Geometry check sheet. Reference: the model listing, model coordinates, mm. Face numbers are marked on the shaded views. A direction names the side the tool comes from. Give positions to 0.01 mm unless a question says otherwise; leave off trailing zeros. Write each loop counter-clockwise with the first axis right and the second up, starting at its lowest first coordinate (ties: lowest second). Pieces come first, ordered by that corner, then holes. Notation, with made-up numbers: (-40, 42) - (19, 42) arc R26 ccw to (19, 78) - close; hole circle Ø4 at (80, -14). An arc over 180 degrees is marked (long way). Write item = value, one per line. Start each with the question number.
(1) Access from +Z, -Z, +X, -X, +Y, -Y to the whole of each face (thin tool, end or side, straight path). Record for the marked faces 4, 5, 6, 7 and 8.
(2) Draft check along X on the marked faces 1, 2 and 3. Enter one of: pulls with the +X half, pulls with the -X half, needs draft (parallel to the pull), parting line crosses it, or undercut.
(3) Section check D-D, the plane z = -0.25. Give the number of separate pieces and of enclosed holes in the cut face, plus the area to 3 significant figures.
(4) Thickness scan on L1, parallel to Y at x = 0, z = 0.5 (3 decimals); L2, parallel to Z at x = -6, y = 10.75 (3 decimals); L3, parallel to Y at x = 0, z = -5 (3 decimals). Record the ranges inside material, lowest first.
(5) Section check A-A, the plane z = -5.5. Enter the section's corners in (x, y) (3 decimals), plus the area to 3 significant figures.
(6) Depth check by flat-ended pin: pin 1 Ø5 at (x, z) = (-13, -7) entering from +Y; pin 2 Ø6.5 at (x, y) = (-2.5, -4.5) entering from +Z (3 decimals); pin 3 Ø5 at (y, z) = (14.5, -2) entering from +X. Enter the tip coordinate at first touch or a pass-through.
(7) Section check B-B, the plane y = 13.5. Enter the section's corners in (x, z) (3 decimals), plus the area to 3 significant figures.
```python
from build123d import *

# Parameters (mm, degrees)
SKETCH1_W           = 38.1
SKETCH1_H           = 19.05
BOSS_EXTRUDE1_DEPTH = 19.05
SKETCH2_R           = 1.5875
CUT_EXTRUDE2_DEPTH  = 19.05
SKETCH3_W           = 16.620070223
SKETCH3_H           = 12.7
CUT_EXTRUDE3_DEPTH  = 19.05
SKETCH4_W           = 12.7
SKETCH4_H           = 12.7
CUT_EXTRUDE4_DEPTH  = 50.8
SKETCH6_W           = 7.660570014
SKETCH6_H           = 3.81
BOSS_EXTRUDE2_DEPTH = 7.62
CUT_EXTRUDE6_DEPTH  = 19.05
SKETCH8_W           = 5.08
SKETCH8_H           = 2.54
BOSS_EXTRUDE3_DEPTH = 2.54
SKETCH9_R           = 0.508
CUT_EXTRUDE7_DEPTH  = 19.05
SKETCH10_W          = 9.525
SKETCH10_H          = 12.7
CUT_EXTRUDE8_DEPTH  = 3.81


with BuildPart() as part:
    # Sketch1 → Boss-Extrude1 (new body)
    with BuildSketch(Plane(origin=(0, 0, 0), x_dir=(1, 0, 0), z_dir=(0, 1, 0))):
        with Locations((-3.175, 0)):
            Rectangle(SKETCH1_W, SKETCH1_H)
    extrude(amount=BOSS_EXTRUDE1_DEPTH)

    # Sketch2 → Cut-Extrude2 (cut)
    with BuildSketch(Plane.XY.offset(9.525)):
        with Locations((-12.7, 9.525)):
            Circle(SKETCH2_R)
        with BuildLine():
            ThreePointArc((-12.7, 19.05), (-22.225, 9.525), (-12.7, 0))
            ThreePointArc((-12.7, 0), (-33.665146333, 9.525), (-12.7, 19.05))
        make_face()
        with BuildLine():
            ThreePointArc((6.35, 0), (15.875, 9.525), (6.35, 19.05))
            ThreePointArc((6.35, 19.05), (24.948138119, 9.525), (6.35, 0))
        make_face()
    extrude(amount=-CUT_EXTRUDE2_DEPTH, mode=Mode.SUBTRACT)

    # Sketch3 → Cut-Extrude3 (cut)
    with BuildSketch(Plane(origin=(0, 19.05, 0), x_dir=(1, 0, 0), z_dir=(0, 1, 0))):
        with Locations((-21.010035112, 0)):
            Rectangle(SKETCH3_W, SKETCH3_H)
    extrude(amount=-CUT_EXTRUDE3_DEPTH, mode=Mode.SUBTRACT)

    # Sketch4 → Cut-Extrude4 (cut)
    with BuildSketch(Plane(origin=(-15.875, 0, 0), x_dir=(0, 0, -1), z_dir=(1, 0, 0))):
        with Locations((0, 9.525)):
            Rectangle(SKETCH4_W, SKETCH4_H)
    extrude(amount=CUT_EXTRUDE4_DEPTH, mode=Mode.SUBTRACT)

    # Sketch6 → Boss-Extrude2 (add)
    with BuildSketch(Plane(origin=(0, 0, 0), x_dir=(1, 0, 0), z_dir=(0, 1, 0))):
        with Locations((-2.519714993, 0)):
            Rectangle(SKETCH6_W, SKETCH6_H)
    extrude(amount=-BOSS_EXTRUDE2_DEPTH)

    # Sketch7 → Cut-Extrude6 (cut)
    with BuildSketch(Plane.XY.offset(9.525)):
        with BuildLine():
            Line((-7.080935196, -3.131729905), (-6.858, 0))
            Line((-6.858, 0), (-6.858, -7.767816491))
            Line((-6.858, -7.767816491), (-14.771031914, -7.767816491))
            Line((-14.771031914, -7.767816491), (-14.771031914, 0))
            Line((-14.771031914, 0), (-9.975013633, 0))
            ThreePointArc((-9.975013633, 0), (-9.162678538, -1.206904896), (-8.794375076, -2.614335284))
            ThreePointArc((-8.794375076, -2.614335284), (-9.25025826, -3.647474967), (-10.163496252, -4.311706442))
            ThreePointArc((-10.163496252, -4.311706442), (-11.221462334, -3.861030674), (-11.89339597, -2.927807191))
            ThreePointArc((-11.89339597, -2.927807191), (-11.604147707, -2.390005207), (-10.996168015, -2.332941862))
            ThreePointArc((-10.996168015, -2.332941862), (-10.54556137, -1.577353268), (-11.301149964, -1.126746624))
            ThreePointArc((-11.301149964, -1.126746624), (-12.52752029, -1.573373178), (-13.044460874, -2.771802103))
            ThreePointArc((-13.044460874, -2.771802103), (-12.016160281, -5.071387383), (-9.595781192, -5.769427237))
            ThreePointArc((-9.595781192, -5.769427237), (-7.890109837, -4.877949662), (-7.080935196, -3.131729905))
        make_face()
        with BuildLine():
            Line((1.563031914, 0), (-3.232986367, 0))
            ThreePointArc((-3.232986367, 0), (-4.045321462, -1.206904896), (-4.413624924, -2.614335284))
            ThreePointArc((-4.413624924, -2.614335284), (-3.95774174, -3.647474967), (-3.044503748, -4.311706442))
            ThreePointArc((-3.044503748, -4.311706442), (-1.986537666, -3.861030674), (-1.31460403, -2.927807191))
            ThreePointArc((-1.31460403, -2.927807191), (-1.603852293, -2.390005207), (-2.211831985, -2.332941862))
            ThreePointArc((-2.211831985, -2.332941862), (-2.66243863, -1.577353268), (-1.906850036, -1.126746624))
            ThreePointArc((-1.906850036, -1.126746624), (-0.68047971, -1.573373178), (-0.163539126, -2.771802103))
            ThreePointArc((-0.163539126, -2.771802103), (-1.191839719, -5.071387383), (-3.612218808, -5.769427237))
            ThreePointArc((-3.612218808, -5.769427237), (-5.317890163, -4.877949662), (-6.127064804, -3.131729905))
            Line((-6.127064804, -3.131729905), (-6.35, 0))
            Line((-6.35, 0), (-6.35, -7.767816491))
            Line((-6.35, -7.767816491), (1.563031914, -7.767816491))
            Line((1.563031914, -7.767816491), (1.563031914, 0))
        make_face()
    extrude(amount=-CUT_EXTRUDE6_DEPTH, mode=Mode.SUBTRACT)

    # Sketch8 → Boss-Extrude3 (add)
    with BuildSketch(Plane(origin=(0, 19.05, 0), x_dir=(1, 0, 0), z_dir=(0, 1, 0))):
        Rectangle(SKETCH8_W, SKETCH8_H)
    extrude(amount=BOSS_EXTRUDE3_DEPTH)

    # Sketch9 → Cut-Extrude7 (cut)
    with BuildSketch(Plane.XY.offset(9.525)):
        with Locations((0, 20.32)):
            Circle(SKETCH9_R)
        with BuildLine():
            ThreePointArc((-2.54, 19.05), (0, 21.59), (2.54, 19.05))
            ThreePointArc((2.54, 19.05), (0, 23.383223271), (-2.54, 19.05))
        make_face()
    extrude(amount=-CUT_EXTRUDE7_DEPTH, mode=Mode.SUBTRACT)

    # Sketch10 → Cut-Extrude8 (cut)
    with BuildSketch(Plane(origin=(0, 19.05, 0), x_dir=(1, 0, 0), z_dir=(0, 1, 0))):
        with Locations((-7.9375, 0)):
            Rectangle(SKETCH10_W, SKETCH10_H)
    extrude(amount=-CUT_EXTRUDE8_DEPTH, mode=Mode.SUBTRACT)


solid = part.part
```
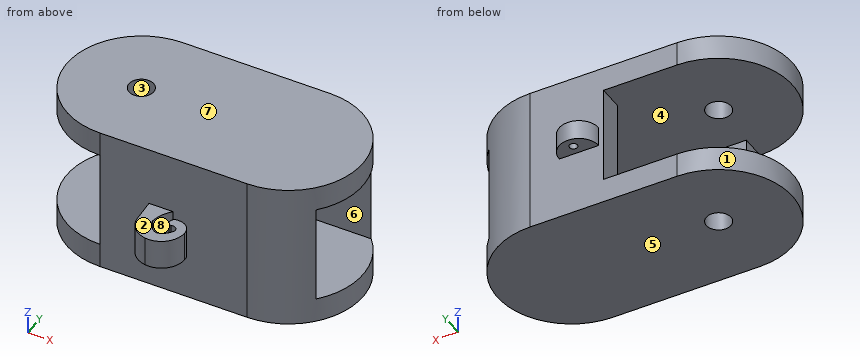
Model answer:
q1.face_4 = -X
q1.face_5 = -Z, +X, -X, +Y, -Y
q1.face_6 = +X, -X
q1.face_7 = +Z, +X, -X, +Y, -Y
q1.face_8 = +Z, -Z
q2.face_1 = pulls with the -X half
q2.face_2 = needs draft
q2.face_3 = undercut
q3.separate_pieces = 2
q3.enclosed_holes = 1
q3.area = 151 mm²
q4.L1 = 0 to 3.175, 15.875 to 19.812, 20.828 to 21.59
q4.L2 = -9.525 to -6.35, 6.35 to 9.525
q4.L3 = 0 to 3.175, 15.875 to 19.05
q5.outline = (-12.7, 0) - (6.35, 0) arc R9.525 ccw to (13.45, 3.175) - (-12.7, 3.175) - close; (-3.175, 15.875) - (13.45, 15.875) arc R9.525 ccw to (6.35, 19.05) - (-3.175, 19.05) - close
q5.area = 122 mm²
q6.pin_1 = 19.05
q6.pin_2 = 1.905
q6.pin_3 = 13.45
q7.outline = (-21.356, -9.525) - (15.006, -9.525) - (15.006, -6.35) - (-21.356, -6.35) - close; (-21.356, 6.35) - (15.006, 6.35) - (15.006, 9.525) - (-21.356, 9.525) - close
q7.area = 231 mm²
